CAD build for the part. Positions are in the model's coordinates, mm. A direction names the side the tool comes from. Give positions to 0.01 mm unless a question says otherwise; leave off trailing zeros. Order: outer loops, then holes, each group sorted by start corner. A loop starts at its lowest first (then second) coordinate and runs counter-clockwise, first axis right, second up.
Item 1: Flat gauge pins, fed straight in: P1, Ø7, axis at x = -20.5, y = -31.5, coming from the -Z side; P2, Ø8, axis at x = -7.5, z = 8, coming from the +Y side; P3, Ø2.5, axis at x = -1, z = 16, coming from the -Y side. Where does each tip first touch, or does it go through?
Item 2: Band-saw the part on B-B on z = 30. Give the cut face in (x, y), plus the area to 3 significant figures.
Item 3: Band-saw the part on D-D on z = 6.5. Give the cut face in (x, y), plus the area to 3 significant figures.
Item 4: Wall check: L1, parallel to X at y = -8, z = 28.5; L2, parallel to Y at x = -34.7, z = 10; L3, parallel to Z at x = -24, y = -33. Give the ranges that are in metal, low to high.
Item 5: Band-saw the part on C-C on y = -22. Give the cut face in (x, z), plus the area to 3 significant figures.
Item 6: Two-plate mould, pull along X, no slides. Class faces 1 (the flat face through (0, -16, 42)), 2 (the flat face through (-1, -11.237, 16)), 3 (the cylindrical face through (-14.1, -15.89, 71.52)): released by +X, released by -X, zero draft, split by the parting line, or undercut.
Item 7: Band-saw the part on A-A on x = -18. Give the cut face in (y, z).
Item 8: Which spindle directions (+Z, -Z, +X, -X, +Y, -Y) get a long thin tool onto all of the face, cutting with end or side? Do faces 4 (the flat face through (-1, -12, 17.013)), 5 (the flat face through (-3, -16, 41)), 6 (the cylindrical face through (-1.479, -20.331, 2.555)). Say none if no direction does.
```python
from build123d import *

# Parameters (mm, degrees)
F1_DEPTH  = 44
F3_DEPTH  = 55.2
F5_DEPTH  = 63.6
F7_DEPTH  = 49.8
F9_DEPTH  = 25
F10_R     = 7.25
F11_DEPTH = 25
F12_R     = 3
F13_R     = 3
F14_R     = 3
F15_R     = 3


with BuildPart() as f1:
    # F0 (on Front) → F1 (new body)
    with BuildSketch(Plane.XZ):
        Polygon((-36, 0), (-33, 0), (-33, 70), (-3, 70), (-3, 0), (0, 0), (0, 73), (-36, 73), align=None)
    extrude(amount=F1_DEPTH)

    # F2 (on face) → F3 (cut)
    with BuildSketch(Plane.YZ):
        Polygon((-44, 73), (-44, 10), (-25.0136986301, 10), align=None)
        Polygon((-25.0136986301, 10), (-44, 10), (-44, 0), (-22, 0), align=None)
    extrude(amount=-F3_DEPTH, mode=Mode.SUBTRACT)

    # F4 (on face) → F5 (cut)
    with BuildSketch(Plane.YZ):
        with BuildLine():
            Line((-24.407023006, 7.9869399744), (-25.0136986301, 10))
            ThreePointArc((-25.0136986301, 10), (-24.7517991178, 8.9809817325), (-24.407023006, 7.9869399744))
        make_face()
        with BuildLine():
            Line((-22, 0), (-14.237880293, 0))
            ThreePointArc((-14.237880293, 0), (-20.4062314251, 2.6135784089), (-24.407023006, 7.9869399744))
            Line((-24.407023006, 7.9869399744), (-22, 0))
        make_face()
        with BuildLine():
            Line((0, 0), (0, 10))
            ThreePointArc((0, 10), (-3.807463773, 3.2969407526), (-10.7758183371, 0))
            Line((-10.7758183371, 0), (0, 0))
        make_face()
    extrude(amount=-F5_DEPTH, mode=Mode.SUBTRACT)

    # F4 (on face) + F6 (on face) → F7 (cut)
    with BuildSketch(Plane.YZ):
        with BuildLine():
            Line((-17.5068493151, 10), (-7.5068493151, 10))
            ThreePointArc((-7.5068493151, 10), (-12.5068493151, 15), (-17.5068493151, 10))
        make_face()
    with BuildSketch(Plane.YZ):
        with BuildLine():
            Line((-7.5068493151, 10), (-17.5068493151, 10))
            ThreePointArc((-17.5068493151, 10), (-12.5068493151, 5), (-7.5068493151, 10))
        make_face()
    extrude(amount=-F7_DEPTH, mode=Mode.SUBTRACT)

    # F8 (on face) → F9 (cut)
    with BuildSketch(Plane.YZ):
        with BuildLine():
            Line((-11.2372876331, 17.0134898722), (-13.7372876331, 17.0134898722))
            Line((-13.7372876331, 17.0134898722), (-13.7372876331, 14.8462378755))
            ThreePointArc((-13.7372876331, 14.8462378755), (-12.4866460858, 14.9999591828), (-11.2372876331, 14.8361361784))
            Line((-11.2372876331, 14.8361361784), (-11.2372876331, 17.0134898722))
        make_face()
        with BuildLine():
            ThreePointArc((-11.2372876331, 14.8361361784), (-12.4866460858, 14.9999591828), (-13.7372876331, 14.8462378755))
            Line((-13.7372876331, 14.8462378755), (-13.7372876331, 13.0134898722))
            Line((-13.7372876331, 13.0134898722), (-11.2372876331, 13.0134898722))
            Line((-11.2372876331, 13.0134898722), (-11.2372876331, 14.8361361784))
        make_face()
    extrude(amount=-F9_DEPTH, mode=Mode.SUBTRACT)

    # F10 (on face) → F11 (cut)
    with BuildSketch(Plane.XY.offset(73)):
        with Locations((-18, -22)):
            Circle(F10_R)
    extrude(amount=-F11_DEPTH, mode=Mode.SUBTRACT)

    # F12
    f12_edges = [f1.edges().sort_by_distance(p)[0] for p in [
        (0, -22, 73),
    ]]
    fillet(f12_edges, radius=F12_R)

    # F13
    f13_edges = [f1.edges().sort_by_distance(p)[0] for p in [
        (-36, -22, 73),
    ]]
    fillet(f13_edges, radius=F13_R)

    # F14
    f14_edges = [f1.edges().sort_by_distance(p)[0] for p in [
        (-33, -21.547945, 70),
    ]]
    fillet(f14_edges, radius=F14_R)

    # F15
    f15_edges = [f1.edges().sort_by_distance(p)[0] for p in [
        (-3, -21.547945, 70),
    ]]
    fillet(f15_edges, radius=F15_R)


solid = f1.part
```
The answers:
1. P1: stops at z = 70
1. P2: passes through
1. P3: stops at y = -27.2
2. outline: (-36, -31.04) - (-33, -31.04) - (-33, 0) - (-36, 0) - close; (-3, -31.04) - (0, -31.04) - (0, 0) - (-3, 0) - close
2. area: 186 mm2
3. outline: (-36, -23.71) - (-33, -23.71) - (-33, -16.08) - (-36, -16.08) - close; (-36, -8.94) - (-33, -8.94) - (-33, -1.31) - (-36, -1.31) - close; (-3, -23.71) - (0, -23.71) - (0, -16.08) - (-3, -16.08) - close; (-3, -8.94) - (0, -8.94) - (0, -1.31) - (-3, -1.31) - close
3. area: 91.6 mm2
4. L1: x = -36 to -33, -3 to 0
4. L2: y = -25.01 to -17.51, -7.51 to 0
4. L3: z = 70 to 73
5. outline: (-36, 4.1) - (-33, 4.1) - (-33, 67) arc R3 cw to (-30, 70) - (-25.25, 70) - (-25.25, 73) - (-33, 73) arc R3 ccw to (-36, 70) - close; (-10.75, 70) - (-6, 70) arc R3 cw to (-3, 67) - (-3, 4.1) - (0, 4.1) - (0, 70) arc R3 ccw to (-3, 73) - (-10.75, 73) - close
5. area: 460 mm2
6. face 1: released by +X
6. face 2: zero draft
6. face 3: undercut
7. outline: (-44, 73) - (-43.1, 70) - (-29.25, 70) - (-29.25, 73) - close; (-14.75, 70) - (0, 70) - (0, 73) - (-14.75, 73) - close
8. face 4: +X
8. face 5: -Z, +Y, -Y
8. face 6: -Z, +X, -X, -Y
